from build123d import *

# Parameters (mm, degrees)
SKETCH1_R           = 11.5
BOSS_EXTRUDE1_DEPTH = 2
CHAMFER1_SIZE       = 1
FILLET2_R           = 0.5


with BuildPart() as part:
    # Sketch1 → Boss-Extrude1 (new body)
    with BuildSketch(Plane.XY):
        Circle(SKETCH1_R)
    extrude(amount=BOSS_EXTRUDE1_DEPTH)

    # Sketch3 → Revolve1 (revolve)
    with BuildSketch(Plane(origin=(0, 0, 0), x_dir=(0, 0, -1), z_dir=(1, 0, 0)), mode=Mode.PRIVATE) as revolve1_sk:
        Polygon((0, 4.5), (0, 6.9), (2.6, 6.9), (2.6, 7.4), (5.6, 5.667949192), (5.6, 4.5), align=None)
    revolve(revolve1_sk.sketch.rotate(Axis((0, 4.5, 0), (0, 0, -1)), 180), axis=Axis((0, 4.5, 0), (0, 0, -1)))

    # Chamfer1
    chamfer1_edges = [part.edges().sort_by_distance(p)[0] for p in [
        (-11.5, 0, 2),
    ]]
    chamfer(chamfer1_edges, length=CHAMFER1_SIZE)

    # Fillet2
    fillet2_edges = [part.edges().sort_by_distance(p)[0] for p in [
        (0, 5.667949192, -5.6),
    ]]
    fillet(fillet2_edges, radius=FILLET2_R)


solid = part.part
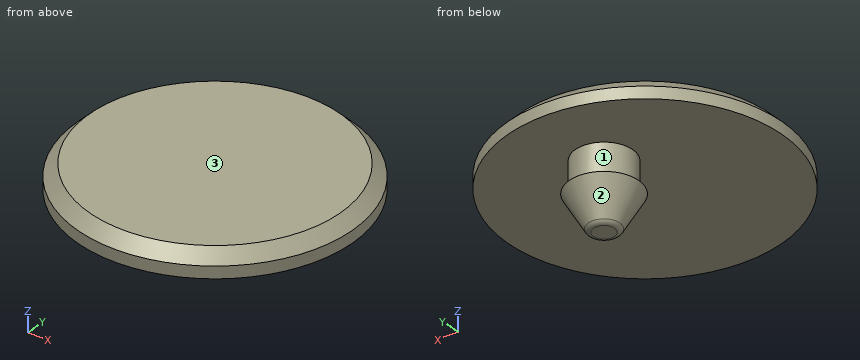
Geometry: final body of the model. Coordinates: model frame, mm. Face numbers are marked on the shaded views. Round coordinates to 2 decimals unless told otherwise and drop trailing zeros. Loops run counter-clockwise (first coordinate to the right, second up) from the corner with the lowest first, then second, coordinate; pieces in that order, holes last.
Q1. Pull-direction query (Z, two-part tool) for the marked faces 1, 2 and 3; classes: released by +Z, released by -Z, zero draft, split by the parting line, or undercut.
Q2. Material intervals for L1, parallel to Z at x = -1, y = -4.75; L2, parallel to Y at x = 2, z = 1.5; L3, parallel to Z at x = 1, y = 3.75, sorted ascending.
Q3. Pin query (flat end, axial travel): P1, Ø2, axis at y = -1.5, z = 0.5, coming from the +X side; P2, Ø11.5, axis at x = -2, y = -3.5, coming from the -Z side; P3, Ø1, axis at y = 6.5, z = 1, coming from the +X side. Return the tip coordinate at first contact, or that it passes through.
Q4. Section A-A on x = 0. Return loops of the section in (y, z), plus the area to 3 significant figures.
Q5. Section C-C on z = -1.25. Return loops of the section in (x, y), plus the area to 3 significant figures.
Q6. Section B-B on y = 0. Return loops of the section in (x, z), plus the area to 3 significant figures.
Evaluation:
1. face 1: undercut
1. face 2: released by -Z
1. face 3: released by +Z
2. L1: z = 0 to 2
2. L2: y = -10.82 to 10.82
2. L3: z = -5.44 to 2
3. P1: stops at x = 11.49
3. P2: stops at z = -3.3
3. P3: stops at x = 9.81
4. outline: (-11.5, 0) - (2.1, 0) - (2.1, -2.6) - (1.6, -2.6) - (3.19, -5.35) arc R0.5 ccw to (3.62, -5.6) - (5.38, -5.6) arc R0.5 ccw to (5.81, -5.35) - (7.4, -2.6) - (6.9, -2.6) - (6.9, 0) - (11.5, 0) - (11.5, 1) - (10.5, 2) - (-10.5, 2) - (-11.5, 1) - close
4. area: 69.7 mm2
5. outline: circle Ø4.8 at (0, 4.5)
5. area: 18.1 mm2
6. outline: (-11.5, 0) - (11.5, 0) - (11.5, 1) - (10.5, 2) - (-10.5, 2) - (-11.5, 1) - close
6. area: 45.0 mm2
